Verification items for this drawing (mm, ordinates from the low corner). A direction names the side the tool comes from. Coordinates: 2 decimals unless noted, no trailing zeros. Order: outer loops, then holes, each group sorted by start corner. A loop starts at its lowest first (then second) coordinate and runs counter-clockwise, first axis right, second up. Notation, with made-up numbers: (71, 81.5) -> (80, 81.5) arc R18 ccw to (80, 104.5) -> close; hole circle Ø6 at (78.25, 71). An arc over 180 degrees is marked (long way). Write item = value, one per line. Start each with the question number.
1. Cross-section at B-B on y = 6.75. Record the cut outline in (x, z) (3 decimals).
2. Cross-section at C-C on x = 9. Record the cut outline in (y, z) (3 decimals), plus the area to 3 significant figures.
3. Thickness scan on line 1 along X through (y, z) = (2.75, 6.5) (3 decimals); line 2 along X through (y, z) = (13.5, 8.75) (3 decimals). Record the ranges inside material, lowest first. Write a range as from..to.
4. Go/stop test with flat-tipped pins: P1, Ø4, axis at x = 12.5, z = 3.5, coming from the +Y side (3 decimals); P2, Ø5, axis at y = 6.5, z = 5.5, coming from the +X side (3 decimals); P3, Ø4, axis at y = 12, z = 9.5, coming from the -X side. Record where each tip stops, or that it passes through.
5. Cross-section at A-A on z = 6.35. Record the cut outline in (x, y) (3 decimals).
6. Set-up check for the marked faces 1 and 2: record each of +Z, -Z, +X, -X, +Y, -Y from which the full face is reachable in a straight line by a thin tool's end or side.
7. Cross-section at D-D on z = 2.25. Record the cut outline in (x, y) (3 decimals).
8. Release check for a two-part mould opening along Y. For the marked faces 3, 4 and 5 record: +Y half, -Y half, draft (parallel to the pull), parting line (faces both ways), or undercut.
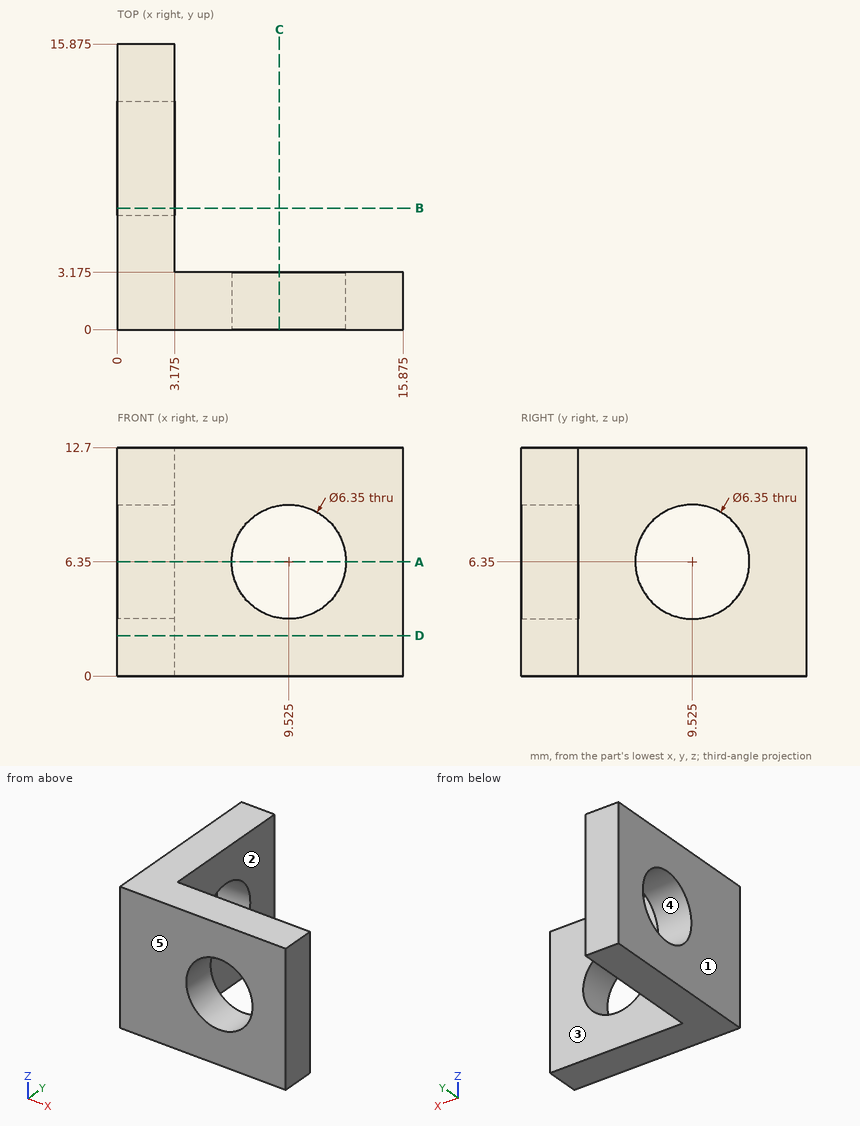
Worked out:
q1.outline = (0, 0) -> (3.175, 0) -> (3.175, 4.807) -> (0, 4.807) -> close; (0, 7.893) -> (3.175, 7.893) -> (3.175, 12.7) -> (0, 12.7) -> close
q2.outline = (0, 0) -> (3.175, 0) -> (3.175, 3.219) -> (0, 3.219) -> close; (0, 9.481) -> (3.175, 9.481) -> (3.175, 12.7) -> (0, 12.7) -> close
q2.area = 20.4 mm²
q3.line_1 = 0..6.354, 12.696..15.875
q3.line_2 = 0..3.175
q4.P1 = 3.175
q4.P2 = 3.175
q4.P3 = 0
q5.outline = (0, 0) -> (6.35, 0) -> (6.35, 3.175) -> (3.175, 3.175) -> (3.175, 6.35) -> (0, 6.35) -> close; (0, 12.7) -> (3.175, 12.7) -> (3.175, 15.875) -> (0, 15.875) -> close; (12.7, 0) -> (15.875, 0) -> (15.875, 3.175) -> (12.7, 3.175) -> close
q6.face_1 = +Z, -Z, -X, +Y, -Y
q6.face_2 = +Z, -Z, +X, +Y
q7.outline = (0, 0) -> (15.875, 0) -> (15.875, 3.175) -> (3.175, 3.175) -> (3.175, 15.875) -> (0, 15.875) -> close
q8.face_3 = +Y half
q8.face_4 = undercut
q8.face_5 = -Y half
